Geometry: final body of the model. Coordinates: model frame, mm. Face numbers are marked on the shaded views. A direction names the side the tool comes from. Round coordinates to 2 decimals unless told otherwise and drop trailing zeros. Loops run counter-clockwise (first coordinate to the right, second up) from the corner with the lowest first, then second, coordinate; pieces in that order, holes last. Notation, with made-up numbers: (-26, -25) - (-18, -25) arc R10 cw to (-18, -15) - close; hole circle Ø9 at (22.25, 20.25). An arc over 180 degrees is marked (long way). Answer as CSV lines item,"result".
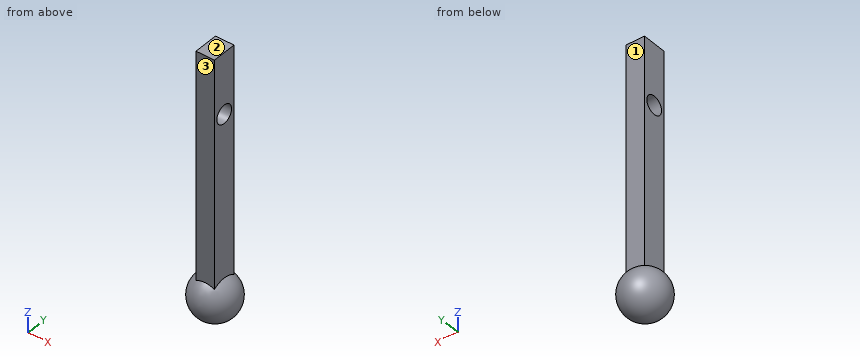
from build123d import *

# Parameters (mm, degrees)
F2_W          = 7.62
F2_H          = 10.1600026736
F3_DEPTH      = 101.6
F4_R          = 3.81
F5_DEPTH      = 9.526
F5_DEPTH_BACK = 9.526


with BuildPart() as f1:
    # F0 (on Right) → F1 (revolve)
    with BuildSketch(Plane.YZ):
        with BuildLine():
            ThreePointArc((0, 9.525), (-9.525, 0), (0, -9.525))
            Line((0, -9.525), (0, 9.525))
        make_face()
    revolve(axis=Axis((0, 0, 0), (0, 0, 1)))

    # F2 (on Top) → F3 (join)
    with BuildSketch(Plane.XY):
        Rectangle(F2_W, F2_H)
    extrude(amount=F3_DEPTH)

    # F4 (on Right) → F5 (cut, two sides)
    with BuildSketch(Plane.YZ) as f5_sk:
        with Locations((0, 76.2)):
            Circle(F4_R)
    extrude(amount=-F5_DEPTH, mode=Mode.SUBTRACT)
    extrude(f5_sk.sketch, amount=F5_DEPTH_BACK, mode=Mode.SUBTRACT)


solid = f1.part
(1) Section C-C (x = 2.25). Output: boundary loops of the cut face in (y, z), and give its area (3 significant figures).
Findings below:
outline,"(-5.08, 7.74) arc R9.26 ccw (long way) to (5.08, 7.74) - (5.08, 101.6) - (-5.08, 101.6) - close; hole circle Ø7.62 at (0, 76.2)"
area,"1,170 mm2"
(2) Section B-B (z = 76.2). Output: boundary loops of the cut face in (x, y), and give its area (3 significant figures).
Findings below:
outline,"(-3.81, -5.08) - (3.81, -5.08) - (3.81, -3.81) - (-3.81, -3.81) - close; (-3.81, 3.81) - (3.81, 3.81) - (3.81, 5.08) - (-3.81, 5.08) - close"
area,"19.4 mm2"
(3) Material intervals for line 1 along Y through (x, z) = (2, 76.2); line 2 along X through (y, z) = (3.5, 86); line 3 along Z through (x, y) = (3.75, 3), sorted ascending.
Findings below:
line 1,"-5.08 to -3.81, 3.81 to 5.08"
line 2,"-3.81 to 3.81"
line 3,"-8.23 to 73.85, 78.55 to 101.6"
(4) Pin query (flat end, axial travel): P1, Ø4, axis at x = 7, y = -2, coming from the +Z side; P2, Ø6, axis at x = -0.5, z = 57.5, coming from the -Y side; P3, Ø6, axis at x = 0.5, z = 36.5, coming from the +Y side. Return the tip coordinate at first contact, or that it passes through.
Findings below:
P1,"z = 7.93"
P2,"y = -5.08"
P3,"y = 5.08"
(5) Access query for the marked faces 1, 2 and 3. Directions: +Z, -Z, +X, -X, +Y, -Y. A direction counts if a zero-diameter tool reaches every point of the face in a straight line with its end or side. Return the directions, or none.
Findings below:
face 1,"+Z, +X, -X, +Y"
face 2,"+Z, +X, -X, +Y, -Y"
face 3,"+Z, +X, -X, -Y"
(6) Section A-A (y = 0). Output: boundary loops of the cut face in (x, z) (3 decimals), and give its area (3 significant figures).
Findings below:
outline,"(-3.81, 8.73) arc R9.525 ccw (long way) to (3.81, 8.73) - (3.81, 72.39) - (-3.81, 72.39) - close; (-3.81, 80.01) - (3.81, 80.01) - (3.81, 101.6) - (-3.81, 101.6) - close"
area,"931 mm2"
(7) Section D-D (z = 52.5). Output: boundary loops of the cut face in (x, y), and give its area (3 significant figures).
Findings below:
outline,"(-3.81, -5.08) - (3.81, -5.08) - (3.81, 5.08) - (-3.81, 5.08) - close"
area,"77.4 mm2"
